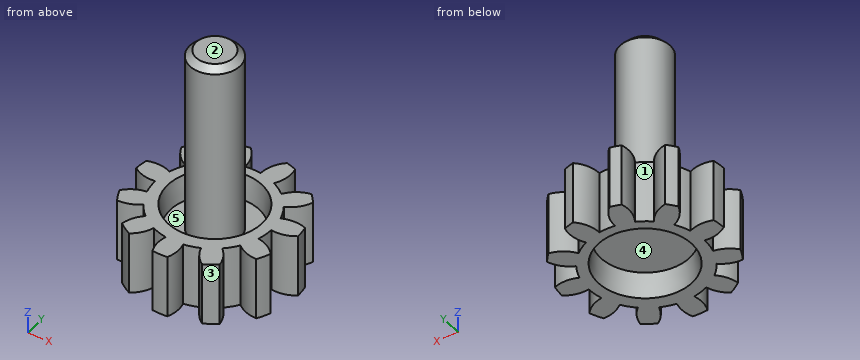
from build123d import *

# Parameters (mm, degrees)
SKETCH_3_R               = 13
EXTRUDE_1_DEPTH          = 10
CUT_EXTRUDE_1_DEPTH      = 21.928449536
PATTERN_CIRCULAR_1_COUNT = 11
SKETCH_5_R               = 7.5
CUT_EXTRUDE_2_DEPTH      = 4
CUT_EXTRUDE_2_DRAFT      = -6
SKETCH_6_R               = 7.5
CUT_EXTRUDE_3_DEPTH      = 4
CUT_EXTRUDE_3_DRAFT      = -6
SKETCH_8_R               = 4
EXTRUDE_3_DEPTH          = 30
CHAMFER_2_SIZE           = 1


with BuildPart() as part:
    # Эскиз3 → Бобышка-Вытянуть1 (new body)
    with BuildSketch(Plane.XY):
        Circle(SKETCH_3_R)
    extrude(amount=-EXTRUDE_1_DEPTH)

    # Эскиз4 → Вырез-Вытянуть1 (cut, through all)
    with BuildSketch(Plane.XY):
        with BuildLine():
            ThreePointArc((2.924363706, 12.666810842), (0, 13), (-2.924363706, 12.666810842))
            ThreePointArc((-2.924363706, 12.666810842), (-1.684886314, 10.969320472), (-1.252557909, 8.912412619))
            ThreePointArc((-1.252557909, 8.912412619), (0, 9), (1.252557909, 8.912412619))
            ThreePointArc((1.252557909, 8.912412619), (1.684886314, 10.969320472), (2.924363706, 12.666810842))
        make_face()
    cut_extrude_1 = extrude(amount=-CUT_EXTRUDE_1_DEPTH, mode=Mode.SUBTRACT)

    # Круговой массив1: Вырез-Вытянуть1 ×11 about axis
    pattern_circular_1_axis = Axis((0, -0.313541407, 0), (0, 0, 1))
    for i in range(1, PATTERN_CIRCULAR_1_COUNT):
        add(cut_extrude_1.rotate(pattern_circular_1_axis, i * 360 / PATTERN_CIRCULAR_1_COUNT), mode=Mode.SUBTRACT)


with BuildPart() as cut_extrude_2_tool:
    # Эскиз5 → Вырез-Вытянуть2 (with draft: the straight prism first)
    with BuildSketch(Plane.XY):
        Circle(SKETCH_5_R)
    extrude(amount=-CUT_EXTRUDE_2_DEPTH)
    # Вырез-Вытянуть2: the draft: its side faces are tilted about the plane it starts from
    cut_extrude_2_sides = [cut_extrude_2_tool.faces().sort_by_distance(p)[0] for p in [
        (-7.5, 0, -2),
    ]]
    draft(cut_extrude_2_sides, Plane.XY, CUT_EXTRUDE_2_DRAFT)


with BuildPart() as part_1:
    add(part.part)

    # Вырез-Вытянуть2: cut by cut_extrude_2_tool
    add(cut_extrude_2_tool.part, mode=Mode.SUBTRACT)


with BuildPart() as cut_extrude_3_tool:
    # Эскиз6 → Вырез-Вытянуть3 (with draft: the straight prism first)
    with BuildSketch(Plane(origin=(0, 0, -10), x_dir=(-1, 0, 0), z_dir=(0, 0, -1))):
        Circle(SKETCH_6_R)
    extrude(amount=-CUT_EXTRUDE_3_DEPTH)
    # Вырез-Вытянуть3: the draft: its side faces are tilted about the plane it starts from
    cut_extrude_3_sides = [cut_extrude_3_tool.faces().sort_by_distance(p)[0] for p in [
        (7.5, 0, -8),
    ]]
    draft(cut_extrude_3_sides, Plane(origin=(0, 0, -10), x_dir=(-1, 0, 0), z_dir=(0, 0, -1)), CUT_EXTRUDE_3_DRAFT)


with BuildPart() as part_2:
    add(part_1.part)

    # Вырез-Вытянуть3: cut by cut_extrude_3_tool
    add(cut_extrude_3_tool.part, mode=Mode.SUBTRACT)

    # Эскиз8 → Бобышка-Вытянуть3 (add)
    with BuildSketch(Plane.XY.offset(-4)):
        Circle(SKETCH_8_R)
    extrude(amount=EXTRUDE_3_DEPTH)

    # Фаска2
    chamfer_2_edges = [part_2.edges().sort_by_distance(p)[0] for p in [
        (-4, 0, 26),
    ]]
    chamfer(chamfer_2_edges, length=CHAMFER_2_SIZE)


solid = part_2.part
For this review, take the finished solid that the model builds, in its own axes (mm). Face numbers are marked on the shaded views. A direction names the side the tool comes from. Give positions to 0.01 mm unless a question says otherwise; leave off trailing zeros. Order: outer loops, then holes, each group sorted by start corner. A loop starts at its lowest first (then second) coordinate and runs counter-clockwise, first axis right, second up. Notation, with made-up numbers: (74, -33) - (83, -33) arc R22 ccw to (83, -21) - close; hole circle Ø11 at (12, -8.75). An arc over 180 degrees is marked (long way). Answer as a JSON object with one key per item and string values. Group by question number.
Item 1: Take a section at A-A on x = 0. Give the boundary of the cut face in (y, z).
Item 2: Take a section at C-C on z = -2. Give the number of separate pieces and of enclosed holes in the cut face, and give its area (3 significant figures).
Item 3: Clearance check with flat-ended pins moving along their axes: pin 1 Ø1.5 at (y, z) = (8, -4.5) entering from -X; pin 2 Ø2 at (x, y) = (8.5, -7) entering from +Z; pin 3 Ø1.5 at (x, z) = (-1, 17) entering from +Y. State where each tip first meets the part, or that it passes through.
Item 4: Wall thickness on line 1 along X through (y, z) = (8.5, -1.5); line 2 along Z through (x, y) = (6.25, -11.25); line 3 along X through (y, z) = (-9.75, -7): over which ranges is each line inside the solid? List them lowest first.
Item 5: Machinability: for the marked faces 4 and 5, which of the approach directions +Z, -Z, +X, -X, +Y, -Y give a long, thin tool a straight path to every point of the face, cutting with its end or side? Answer none if there is none.
Item 6: Draft analysis for pull direction Y (two halves, no side actions). For the marked faces 1, 2 and 3, state which applies: pulls with the +Y half, pulls with the -Y half, needs draft (parallel to the pull), parting line crosses it, or undercut.
Item 7: Take a section at B-B on z = 13. Give the boundary of the cut face in (x, y), and give its area (3 significant figures).
Reported:
{
 "1": {"outline": "(-13, -10) - (-7.5, -10) - (-7.08, -6) - (7.08, -6) - (7.5, -10) - (9, -10) - (9, 0) - (7.5, 0) - (7.08, -4) - (4, -4) - (4, 25) - (3, 26) - (-3, 26) - (-4, 25) - (-4, -4) - (-7.08, -4) - (-7.5, 0) - (-13, 0) - close"},
 "2": {"separate pieces": "2", "enclosed holes": "1", "area": "275 mm^2"},
 "3": {"pin 1": "x = -10.55", "pin 2": "z = 0", "pin 3": "y = 3.99"},
 "4": {"line 1": "-9.84 to -7.91, -4.16 to 4.16, 7.91 to 9.84", "line 2": "-10 to 0", "line 3": "-7.71 to -4.18, -1.46 to 1.46, 4.18 to 7.71"},
 "5": {"face 4": "-Z", "face 5": "+Z"},
 "6": {"face 1": "undercut", "face 2": "needs draft", "face 3": "pulls with the -Y half"},
 "7": {"outline": "circle Ø8 at (0, 0)", "area": "50.3 mm^2"}
}
